The listing builds one solid part. Answer for the finished solid, in the listing's coordinates (mm). Face numbers are marked on the shaded views. A direction names the side the tool comes from. Coordinates: 2 decimals unless noted, no trailing zeros. Order: outer loops, then holes, each group sorted by start corner. A loop starts at its lowest first (then second) coordinate and runs counter-clockwise, first axis right, second up. Notation, with made-up numbers: (1.25, 49.25) - (46.25, 49.25) arc R25 ccw to (46.25, 71.25) - close; hole circle Ø11 at (-34, -20.75). An arc over 180 degrees is marked (long way). Use one line per item in the form item = value. Start each with the question number.
Item 1: Section A-A, the plane x = 96 is taken. Write down the section's boundary in (y, z).
Item 2: Consider line 1 along Y through (x, z) = (134.5, 0.5); line 2 along X through (y, z) = (6.25, 0.25); line 3 along Z through (x, y) = (135, -3.5). Determine where each line is inside the solid, lowest interval first. Write a range as [from, to].
Item 3: Section B-B, the plane x = 16 is taken. Write down the section's boundary in (y, z).
Item 4: Each of these flat-tipped pins is pushed along its axis until it touches: pin 1 Ø1.5 at (x, y) = (60.5, -3) entering from -Z; pin 2 Ø4 at (x, z) = (82, -5) entering from +Y; pin 3 Ø2 at (x, y) = (64.5, -3.5) entering from +Z; pin 4 Ø7.5 at (y, z) = (-2.5, 2) entering from -X. Where does it stop, or does it pass through?
Item 5: A tool of negligible diameter and unlimited length cuts with its end or side. For the marked faces 1, 2 and 3, from which of +Z, -Z, +X, -X, +Y, -Y can it reach the whole face along a straight path? Write none if from no direction.
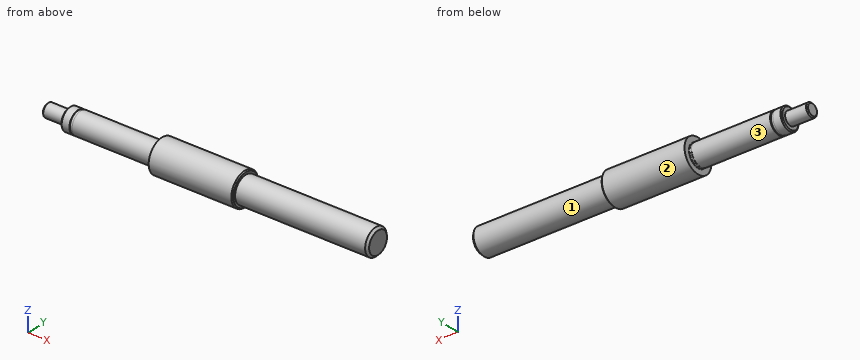
from build123d import *
from build123d.topology import SkipClean

# Parameters (mm, degrees)
SKIZZE1_W = 1.055662433
SKIZZE1_H = 4.75


with BuildPart() as part:
    # Skizze1 → Rotation1 (revolve)
    with SkipClean():  # the faces are left unmerged after this step: merging them gives an invalid solid
        with BuildSketch(Plane(origin=(0, 0, 0), x_dir=(1, 0, 0), z_dir=(0, 1, 0))):
            Polygon((3, 0), (-7, 0), (-7, -2.5), (-6.5, -3), (3, -3), align=None)
            Polygon((-7, 2.5), (-7, 0), (3, 0), (3, 3), (-6.5, 3), align=None)
            Polygon((7, 0), (3, 0), (3, -3), (3, -4.5), (3.5, -5), (7, -5), (7, -4.75), align=None)
            Polygon((3, 3), (3, 0), (7, 0), (7, 4.75), (7, 5), (3.5, 5), (3, 4.5), align=None)
            with Locations((7.527831217, 2.375)):
                Rectangle(SKIZZE1_W, SKIZZE1_H)
            with Locations((7.527831217, -2.375)):
                Rectangle(SKIZZE1_W, SKIZZE1_H)
            Polygon((8.055662433, 4.75), (8.055662433, 0), (8.2, 0), (8.2, 5), align=None)
            Polygon((8.2, 0), (8.055662433, 0), (8.055662433, -4.75), (8.2, -5), align=None)
            with BuildLine():
                Line((8.2, 5), (8.2, 0))
                Line((8.2, 0), (45, 0))
                Line((45, 0), (45, 5.15))
                ThreePointArc((45, 5.15), (44.912132034, 4.937867966), (44.7, 4.85))
                Line((44.7, 4.85), (44.082842712, 4.85))
                ThreePointArc((44.082842712, 4.85), (44.006306026, 4.865224093), (43.941421356, 4.908578644))
                Line((43.941421356, 4.908578644), (43.85, 5))
                Line((43.85, 5), (8.2, 5))
            make_face()
            with BuildLine():
                Line((45, 0), (8.2, 0))
                Line((8.2, 0), (8.2, -5))
                Line((8.2, -5), (43.85, -5))
                Line((43.85, -5), (43.941421356, -4.908578644))
                ThreePointArc((43.941421356, -4.908578644), (44.006306026, -4.865224093), (44.082842712, -4.85))
                Line((44.082842712, -4.85), (44.7, -4.85))
                ThreePointArc((44.7, -4.85), (44.912132034, -4.937867966), (45, -5.15))
                Line((45, -5.15), (45, 0))
            make_face()
            Polygon((45, 5.15), (45, 0), (65, 0), (83, 0), (83, 6), (83, 7), (82.5, 7.5), (45, 7.5), align=None)
            Polygon((65, 0), (45, 0), (45, -5.15), (45, -7.5), (82.5, -7.5), (83, -7), (83, -6), (83, 0), align=None)
            Polygon((143, 0), (83, 0), (83, -6), (142, -6), (143, -5), align=None)
            Polygon((83, 6), (83, 0), (143, 0), (143, 5), (142, 6), align=None)
        revolve(axis=Axis((65, 0, 0), (1, 0, 0)))
    add(part.part.scale(1), mode=Mode.REPLACE)  # the faces are merged on a copy


solid = part.part
Response:
q1.outline = circle Ø12 at (0, 0)
q2.line_1 = [-5.98, 5.98]
q2.line_2 = [45, 83]
q2.line_3 = [-4.87, 4.87]
q3.outline = circle Ø10 at (0, 0)
q4.pin_1 = -7.15
q4.pin_2 = 6.87
q4.pin_3 = 7.07
q4.pin_4 = -7
q5.face_1 = +X
q5.face_2 = +X, -X
q5.face_3 = -X
